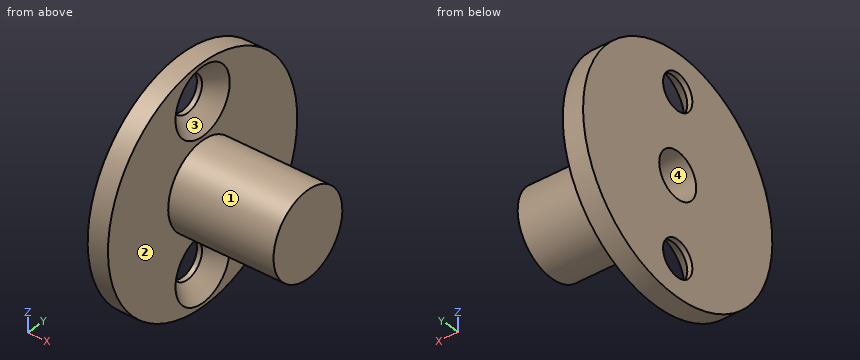
from build123d import *

# Parameters (mm, degrees)
SKETCH1_R                                      = 11
SKETCH1_R_2                                    = 1.6
BOSS_EXTRUDE1_DEPTH                            = 1.93
SKETCH2_R                                      = 4
BOSS_EXTRUDE2_DEPTH                            = 10
SKETCH3_R                                      = 2.15
CUT_EXTRUDE1_DEPTH                             = 6
CSK_FOR_M3_FLAT_HEAD_MACHINE_SCREW1_AT_2_COUNT = 2
CSK_FOR_M3_FLAT_HEAD_MACHINE_SCREW1_AT_2_PITCH = 15


with BuildPart() as part:
    # Sketch1 → Boss-Extrude1 (new body)
    with BuildSketch(Plane(origin=(0, 0, 0), x_dir=(0, 0, -1), z_dir=(1, 0, 0))):
        Circle(SKETCH1_R)
        with Locations((7.5, 0)):
            Circle(SKETCH1_R_2, mode=Mode.SUBTRACT)
        with Locations((-7.5, 0)):
            Circle(SKETCH1_R_2, mode=Mode.SUBTRACT)
    extrude(amount=BOSS_EXTRUDE1_DEPTH)

    # Sketch2 → Boss-Extrude2 (add)
    with BuildSketch(Plane(origin=(1.93, 0, 0), x_dir=(0, 0, -1), z_dir=(1, 0, 0))):
        Circle(SKETCH2_R)
    extrude(amount=BOSS_EXTRUDE2_DEPTH)

    # Sketch3 → Cut-Extrude1 (cut)
    with BuildSketch(Plane(origin=(0, 0, 0), x_dir=(0, 0, -1), z_dir=(1, 0, 0))):
        Circle(SKETCH3_R)
    extrude(amount=CUT_EXTRUDE1_DEPTH, mode=Mode.SUBTRACT)

    # Sketch5 → CSK for M3 Flat Head Machine Screw1 (revolve, cut)
    with BuildSketch(Plane(origin=(1.93, 0, 7.5), x_dir=(0, 0, -1), z_dir=(0, 1, 0))):
        Polygon((0, 0), (0, 1.93), (1.7, 1.93), (1.7, 1.45), (3.15, 0), align=None)
    csk_for_m3_flat_head_machine_screw1 = revolve(axis=Axis((8.28, 0, 7.5), (-1, 0, 0)), mode=Mode.SUBTRACT)

    # CSK for M3 Flat Head Machine Screw1 at 2: CSK for M3 Flat Head Machine Screw1 ×2
    with Locations(*[(0, 0, -i * CSK_FOR_M3_FLAT_HEAD_MACHINE_SCREW1_AT_2_PITCH) for i in range(1, CSK_FOR_M3_FLAT_HEAD_MACHINE_SCREW1_AT_2_COUNT)]):
        add(csk_for_m3_flat_head_machine_screw1, mode=Mode.SUBTRACT)


solid = part.part
Can you work these out from the model? Positions are in its coordinate system, mm. Face numbers are marked on the shaded views. Give positions to 0.01 mm unless a question says otherwise; leave off trailing zeros. Loops run counter-clockwise (first coordinate to the right, second up) from the corner with the lowest first, then second, coordinate; pieces in that order, holes last. Notation, with made-up numbers: (-24, -8) -> (34, -8) arc R25 ccw to (34, 27) -> close; hole circle Ø3 at (43, -32.75). An arc over 180 degrees is marked (long way). Use one line per item in the form item = value.
1) I need wall thicknesses on line 1 along Y through (x, z) = (2.85, 0); line 2 along X through (y, z) = (8, -0.5); line 3 along Y through (x, z) = (0.4, 7.5). Which ranges of each line are inside material? Lowest first, please.
Answers:
line_1 = -4 to -2.15, 2.15 to 4
line_2 = 0 to 1.93
line_3 = -8.05 to -1.7, 1.7 to 8.05
2) If we section it at B-B (z = 7.5): Please give me the cut outline in (x, y).
Answers:
outline = (0, -8.05) -> (1.93, -8.05) -> (1.93, -3.15) -> (0.48, -1.7) -> (0, -1.7) -> close; (0, 1.7) -> (0.48, 1.7) -> (1.93, 3.15) -> (1.93, 8.05) -> (0, 8.05) -> close
3) If we section it at C-C (x = 4.5): Please give me the cut outline in (y, z).
Answers:
outline = circle Ø8 at (0, 0); hole circle Ø4.3 at (0, 0)
4) Will these pins go through, and if not, where does the flat tip stop? pin 1 (1.5 mm diameter, centred on y = -7, z = -7.5, fed in from +X); pin 2 (3.5 mm diameter, centred on y = -0.5, z = 0.5, fed in from -X); pin 3 (3 mm diameter, centred on x = 9.5, z = 2, fed in from +Y); pin 4 (4 mm diameter, centred on y = 0, z = 7.5, fed in from +X).
Answers:
pin_1 = 1.93
pin_2 = 0
pin_3 = 3.97
pin_4 = 0.78
5) If we section it at D-D (x = 1): Please give me the cut outline in (y, z).
Answers:
outline = circle Ø22 at (0, 0); hole circle Ø4.44 at (0, -7.5); hole circle Ø4.44 at (0, 7.5); hole circle Ø4.3 at (0, 0)
6) We'd pull the mould along Z, two halves only. Please class the marked faces 1, 2, 3 and 4: released by +Z, released by -Z, zero draft, split by the parting line, or undercut.
Answers:
face_1 = split by the parting line
face_2 = zero draft
face_3 = undercut
face_4 = undercut
7) If we section it at A-A (y = 0): Please give me the cut outline in (x, z).
Answers:
outline = (0, -11) -> (1.93, -11) -> (1.93, -10.65) -> (0.48, -9.2) -> (0, -9.2) -> close; (0, -5.8) -> (0.48, -5.8) -> (1.93, -4.35) -> (1.93, -4) -> (11.93, -4) -> (11.93, 4) -> (1.93, 4) -> (1.93, 4.35) -> (0.48, 5.8) -> (0, 5.8) -> (0, 2.15) -> (6, 2.15) -> (6, -2.15) -> (0, -2.15) -> close; (0, 9.2) -> (0.48, 9.2) -> (1.93, 10.65) -> (1.93, 11) -> (0, 11) -> close
